For this review, take the finished solid that the model builds, in its own axes (mm). A direction names the side the tool comes from. Round coordinates to 2 decimals unless told otherwise and drop trailing zeros. Write each loop counter-clockwise with the first axis right and the second up, starting at its lowest first coordinate (ties: lowest second). Pieces come first, ordered by that corner, then holes. Notation, with made-up numbers: M 70,-13.5 L 119,-13.5 A22 ccw 119,18.5 Z; hole C 66.25,-13.75 d3. An arc over 180 degrees is marked long. One line per question, with ' | ' between items.
```python
from build123d import *

# Parameters (mm, degrees)
SKETCH1_W            = 155.956
SKETCH1_H            = 68.320954018
BOSS_EXTRUDE1_DEPTH  = 4.5085
SKETCH2_W            = 155.956
SKETCH2_H            = 15.933454036
CUT_EXTRUDE1_DEPTH   = 10.795
BOSS_EXTRUDE2_DEPTH  = 4.5085
CUT_EXTRUDE2_DEPTH   = 4.7625
LPATTERN1_COUNT      = 3
LPATTERN1_PITCH      = 39.916133528
CUT_EXTRUDE3_DEPTH   = 4.7625
FILLET2_R            = 1.905
MIRROR3_COPY_1_DEPTH = 4.7625
MIRROR3_COPY_2_DEPTH = 4.7625
MIRROR3_COPY_3_DEPTH = 4.7625
FILLET3_R            = 1.905
CHAMFER1_SIZE        = 6.35


with BuildPart() as part:
    # Sketch1 → Boss-Extrude1 (new body)
    with BuildSketch(Plane.XY):
        Rectangle(SKETCH1_W, SKETCH1_H)
    extrude(amount=BOSS_EXTRUDE1_DEPTH)

    # Sketch2 → Cut-Extrude1 (cut)
    with BuildSketch(Plane.XY.offset(4.5085)):
        with Locations((0, 26.193749991)):
            Rectangle(SKETCH2_W, SKETCH2_H)
    extrude(amount=-CUT_EXTRUDE1_DEPTH, mode=Mode.SUBTRACT)

    # Sketch3 → Boss-Extrude2 (add)
    with BuildSketch(Plane.XY.offset(4.5085)):
        Polygon((-77.978, -29.334477009), (-87.63, -29.334477009), (-87.63, -25.589053013), (-87.63, -11.808477009), (-82.804, -11.808477009), (-82.804, -24.508477009), (-77.978, -24.508477009), align=None)
        Polygon((-77.978, 10.543522991), (-87.63, 10.543522991), (-87.63, 28.069522991), (-82.804, 28.069522991), (-82.804, 15.369522991), (-77.978, 15.369522991), align=None)
    boss_extrude2 = extrude(amount=-BOSS_EXTRUDE2_DEPTH)

    # Mirror1: Boss-Extrude2 across plane
    add(boss_extrude2.mirror(Plane(origin=(0, 0, 0), x_dir=(0, 0, 1), z_dir=(1, 0, 0))))

    # Sketch4 → Cut-Extrude2 (cut)
    with BuildSketch(Plane(origin=(0, 0, 0), x_dir=(-1, 0, 0), z_dir=(0, 0, -1))):
        Polygon((-74.803, 15.052022991), (-55.753, 15.052022991), (-65.278, -3.997977009), align=None)
    cut_extrude2 = extrude(amount=-CUT_EXTRUDE2_DEPTH, mode=Mode.SUBTRACT)

    # LPattern1: Cut-Extrude2 ×3
    with Locations(*[(-i * LPATTERN1_PITCH, 0, 0) for i in range(1, LPATTERN1_COUNT)]):
        add(cut_extrude2, mode=Mode.SUBTRACT)

    # Sketch5 → Cut-Extrude3 (cut)
    with BuildSketch(Plane(origin=(0, 0, 0), x_dir=(-1, 0, 0), z_dir=(0, 0, -1))):
        Polygon((-52.578, 15.052022991), (-38.061866472, 15.052022991), (-28.536866472, -3.997977009), (-62.103, -3.997977009), align=None)
    cut_extrude3 = extrude(amount=-CUT_EXTRUDE3_DEPTH, mode=Mode.SUBTRACT)

    # Mirror2: Cut-Extrude3 across plane
    add(cut_extrude3.mirror(Plane(origin=(0, 0, 0), x_dir=(0, 0, 1), z_dir=(1, 0, 0))), mode=Mode.SUBTRACT)

    # Fillet2
    fillet2_edges = [part.edges().sort_by_distance(p)[0] for p in [
        (65.278, -3.997977009, 2.25425),
        (74.803, 15.052022991, 2.25425),
        (55.753, 15.052022991, 2.25425),
        (25.361866472, -3.997977009, 2.25425),
        (34.886866472, 15.052022991, 2.25425),
        (15.836866472, 15.052022991, 2.25425),
        (-5.029267056, 15.052022991, 2.25425),
        (-14.554267056, -3.997977009, 2.25425),
        (-24.079267056, 15.052022991, 2.25425),
    ]]
    fillet(fillet2_edges, radius=FILLET2_R)

    # Mirror3: Cut-Extrude2, Cut-Extrude3 across plane
    add(cut_extrude2.mirror(Plane.ZX.offset(-7.966727018)), mode=Mode.SUBTRACT)
    add(cut_extrude3.mirror(Plane.ZX.offset(-7.966727018)), mode=Mode.SUBTRACT)

    # Mirror3 copy 1 sketch → Mirror3 copy 1 (cut)
    with BuildSketch(Plane(origin=(-39.916133528, -15.933454036, 0), x_dir=(-1, 0, 0), z_dir=(0, 0, -1))):
        Polygon((-74.803, -15.052022991), (-55.753, -15.052022991), (-65.278, 3.997977009), align=None)
    extrude(amount=-MIRROR3_COPY_1_DEPTH, mode=Mode.SUBTRACT)

    # Mirror3 copy 2 sketch → Mirror3 copy 2 (cut)
    with BuildSketch(Plane(origin=(-79.832267056, -15.933454036, 0), x_dir=(-1, 0, 0), z_dir=(0, 0, -1))):
        Polygon((-74.803, -15.052022991), (-55.753, -15.052022991), (-65.278, 3.997977009), align=None)
    extrude(amount=-MIRROR3_COPY_2_DEPTH, mode=Mode.SUBTRACT)

    # Mirror3 copy 3 sketch → Mirror3 copy 3 (cut)
    with BuildSketch(Plane(origin=(0, -15.933454036, 0), x_dir=(1, 0, 0), z_dir=(0, 0, -1))):
        Polygon((-52.578, 15.052022991), (-38.061866472, 15.052022991), (-28.536866472, -3.997977009), (-62.103, -3.997977009), align=None)
    extrude(amount=-MIRROR3_COPY_3_DEPTH, mode=Mode.SUBTRACT)

    # Fillet3
    fillet3_edges = [part.edges().sort_by_distance(p)[0] for p in [
        (62.103, -3.997977009, 2.25425),
        (52.578, 15.052022991, 2.25425),
        (38.061866472, 15.052022991, 2.25425),
        (28.536866472, -3.997977009, 2.25425),
        (-52.578, 15.052022991, 2.25425),
        (-62.103, -3.997977009, 2.25425),
        (-28.536866472, -3.997977009, 2.25425),
        (-38.061866472, 15.052022991, 2.25425),
        (74.803, -30.985477027, 2.25425),
        (65.278, -11.935477027, 2.25425),
        (55.753, -30.985477027, 2.25425),
        (34.886866472, -30.985477027, 2.25425),
        (25.361866472, -11.935477027, 2.25425),
        (15.836866472, -30.985477027, 2.25425),
        (-5.029267056, -30.985477027, 2.25425),
        (-14.554267056, -11.935477027, 2.25425),
        (-24.079267056, -30.985477027, 2.25425),
        (-62.103, -11.935477027, 2.25425),
        (-52.578, -30.985477027, 2.25425),
        (-38.061866472, -30.985477027, 2.25425),
        (-28.536866472, -11.935477027, 2.25425),
        (52.578, -30.985477027, 2.25425),
        (62.103, -11.935477027, 2.25425),
        (28.536866472, -11.935477027, 2.25425),
        (38.061866472, -30.985477027, 2.25425),
    ]]
    fillet(fillet3_edges, radius=FILLET3_R)

    # Chamfer1
    # the kernel refuses this chamfer: 6.35 mm, written as the material it adds along each edge
    with BuildSketch(Plane(origin=(-77.978, -29.334477009, 4.5085), x_dir=(-0.9996219169112966, 0.027495876610585696, 0), z_dir=(0, 0, -1))) as chamfer1_piece_1_section:
        Polygon((CHAMFER1_SIZE * 0.999621916911, -CHAMFER1_SIZE * 0.0274958766106), (-CHAMFER1_SIZE * 0.0274958766106, -CHAMFER1_SIZE * 0.999621916911), (0, 0), align=None)
    chamfer1_piece_1 = extrude(amount=4.5085, mode=Mode.PRIVATE)
    chamfer1_piece_1 = split(chamfer1_piece_1, bisect_by=Plane(origin=(-80.204608327, -34.160477009, 2.25425), z_dir=(0, 1, 0)), keep=Keep.TOP, mode=Mode.PRIVATE)
    add(chamfer1_piece_1)
    with BuildSketch(Plane(origin=(-77.978, 10.543522991, 4.5085), x_dir=(-0.9996219169112966, 0.02749587661058624, 0), z_dir=(0, 0, -1))) as chamfer1_piece_2:
        Polygon((CHAMFER1_SIZE * 0.999621916911, -CHAMFER1_SIZE * 0.0274958766106), (-CHAMFER1_SIZE * 0.0274958766106, -CHAMFER1_SIZE * 0.999621916911), (0, 0), align=None)
    extrude(amount=4.5085)
    with BuildSketch(Plane(origin=(77.978, -29.334477009, 4.5085), x_dir=(0.9996219169112966, 0.027495876610585696, 0), z_dir=(0, 0, -1))) as chamfer1_piece_3_section:
        Polygon((CHAMFER1_SIZE * 0.999621916911, CHAMFER1_SIZE * 0.0274958766106), (-CHAMFER1_SIZE * 0.0274958766106, CHAMFER1_SIZE * 0.999621916911), (0, 0), align=None)
    chamfer1_piece_3 = extrude(amount=4.5085, mode=Mode.PRIVATE)
    chamfer1_piece_3 = split(chamfer1_piece_3, bisect_by=Plane(origin=(80.204608327, -34.160477009, 2.25425), z_dir=(0, 1, 0)), keep=Keep.TOP, mode=Mode.PRIVATE)
    add(chamfer1_piece_3)
    with BuildSketch(Plane(origin=(77.978, 10.543522991, 4.5085), x_dir=(0.9996219169112966, 0.027495876610585966, 0), z_dir=(0, 0, -1))) as chamfer1_piece_4:
        Polygon((CHAMFER1_SIZE * 0.999621916911, CHAMFER1_SIZE * 0.0274958766106), (-CHAMFER1_SIZE * 0.0274958766106, CHAMFER1_SIZE * 0.999621916911), (0, 0), align=None)
    extrude(amount=4.5085)


solid = part.part
```
Item 1: Mouldability with a two-part tool opening along X and no side actions: class faces 1 (the face through (33.78, -22.42, 2.22)), 2 (the face through (-80, -24.508, 2)), 3 (the face through (85, -11.808, 2)), 4 (the face through (-87.63, 19, 2)) as +X half, -X half, draft (parallel to the pull), parting line (faces both ways), or undercut.
Results:
face 1: undercut | face 2: undercut | face 3: draft | face 4: -X half
Item 2: Insertion check: pin 1 Ø1.4 at (x, z) = (-81.5, 2) entering from +Y; pin 2 Ø2 at (y, z) = (-5.5, 3.5) entering from -X; pin 3 Ø1 at (x, z) = (85.5, 2.5) entering from -Y. Each pin has a flat end and moves straight along its axis. Give the tip position at first contact, or say it passes through.
Results:
pin 1: y = 15.37 | pin 2: x = -77.98 | pin 3: y = -29.33
Item 3: Take a section at A-A (y = -21). State how many separate pieces and enclosed holes the cut face has, then the cut area to 3 significant figures.
Results:
separate pieces: 8 | enclosed holes: 0 | area: 403 mm2
Item 4: Take a section at B-B (x = -4). Write out the cut boundary in (y, z), then the cut area to 3 significant figures.
Results:
outline: M -34.16,0 L 18.23,0 L 18.23,4.51 L -34.16,4.51 Z | area: 236 mm2
Item 5: To check wall thickness, follow line 1 along X through (y, z) = (-14, 3.4); line 2 along Y through (x, z) = (-42, 2.7); line 3 along X through (y, z) = (17.5, 0.4). State the ranges of each line that lie inside material, in increasing order. Write a range as from..to.
Results:
line 1: -87.63..-82.8, -77.98..-60.92, -29.72..29.72, 60.92..77.98, 82.8..87.63 | line 2: -34.16..-30.99, -11.94..-4, 15.05..18.23 | line 3: -87.63..-82.8, -77.98..77.98, 82.8..87.63
Item 6: Machinability: for faces 5 (the face through (-86, -29.334, 2)), 6 (the face through (-14, -30.985, 2)), 7 (the face through (-80, 15.37, 2)), which of the approach directions +Z, -Z, +X, -X, +Y, -Y give a long, thin tool a straight path to every point of the face, cutting with its end or side? Answer none if there is none.
Results:
face 5: +Z, -Z, -X, -Y | face 6: +Z, -Z | face 7: +Z, -Z, +Y
